Input: dimensioned drawing with shaded views. Units: mm. Origin: part minimum x, y, z. Round coordinates to 2 decimals unless told otherwise and drop trailing zeros. Write each loop counter-clockwise with the first axis right and the second up, starting at its lowest first coordinate (ties: lowest second). Pieces come first, ordered by that corner, then holes. Notation, with made-up numbers: (61, 12) - (80, 12) arc R27 ccw to (80, 36) - close; hole circle Ø8 at (5, 73.25). An arc over 180 degrees is marked (long way). Use one line per item in the form item = value.
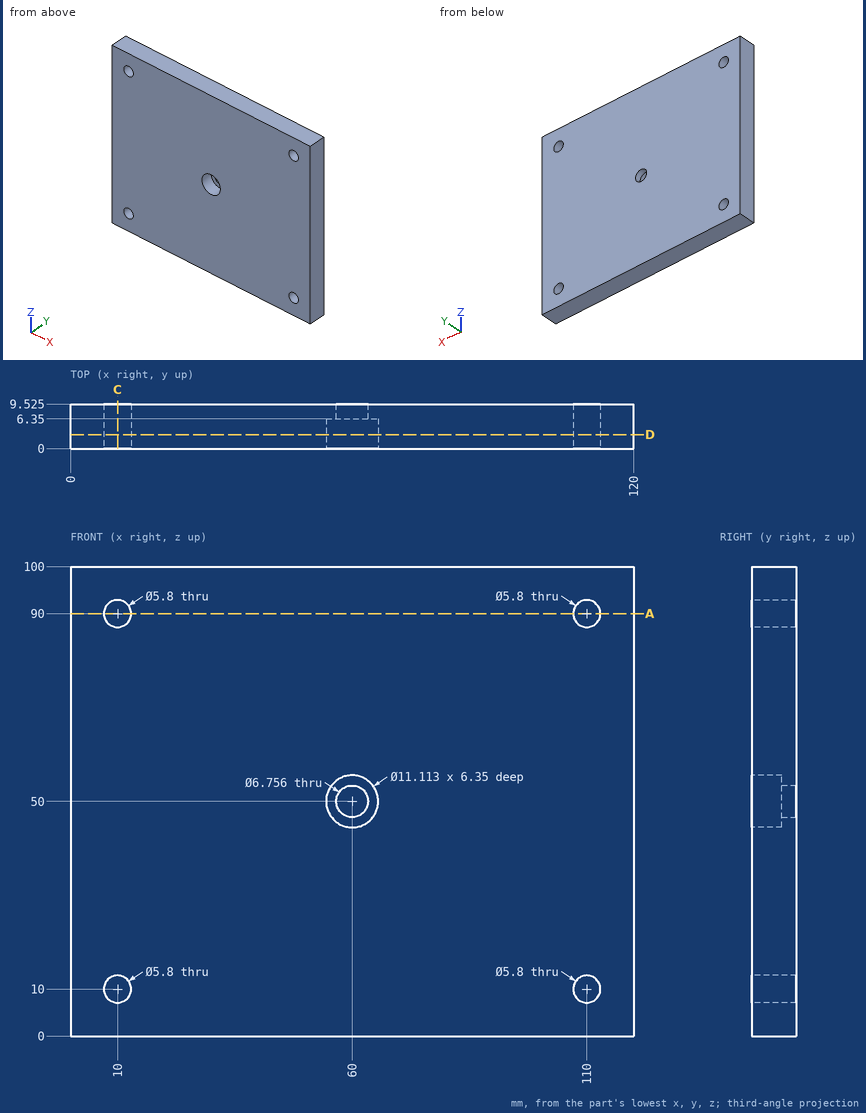
(1) Cut plane D-D on y = 3. Output: boundary loops of the cut face in (x, z).
Derived:
outline = (0, 0) - (120, 0) - (120, 100) - (0, 100) - close; hole circle Ø5.8 at (10, 10); hole circle Ø5.8 at (10, 90); hole circle Ø11.11 at (60, 50); hole circle Ø5.8 at (110, 10); hole circle Ø5.8 at (110, 90)
(2) Cut plane C-C on x = 10. Output: boundary loops of the cut face in (y, z) (1 decimal).
Derived:
outline = (0, 0) - (9.5, 0) - (9.5, 7.1) - (0, 7.1) - close; (0, 12.9) - (9.5, 12.9) - (9.5, 87.1) - (0, 87.1) - close; (0, 92.9) - (9.5, 92.9) - (9.5, 100) - (0, 100) - close
(3) Material intervals for L1, parallel to X at y = 3.75, z = 10; L2, parallel to Z at x = 110, y = 3; L3, parallel to X at y = 8, z = 50, sorted ascending.
Derived:
L1 = 0 to 7.1, 12.9 to 107.1, 112.9 to 120
L2 = 0 to 7.1, 12.9 to 87.1, 92.9 to 100
L3 = 0 to 56.62, 63.38 to 120
(4) Cut plane A-A on z = 90. Output: boundary loops of the cut face in (x, y) (1 decimal).
Derived:
outline = (0, 0) - (7.1, 0) - (7.1, 9.5) - (0, 9.5) - close; (12.9, 0) - (107.1, 0) - (107.1, 9.5) - (12.9, 9.5) - close; (112.9, 0) - (120, 0) - (120, 9.5) - (112.9, 9.5) - close
(5) First-contact query: pin 1 Ø5 at (x, z) = (10, 10) entering from -Y (3 decimals). Flat tip, straight axial feed; report the tip coordinate or a pass-through.
Derived:
pin_1 = through
